from build123d import *

# Parameters (mm, degrees)
BOSS_EXTRUDE1_DEPTH = 3.1242
FILLET4_R           = 12.7
FILLET8_R           = 1.5875
FILLET9_R           = 3.175
CUT_EXTRUDE1_DEPTH  = 116.691473387
SKETCH3_R           = 1.5
CUT_EXTRUDE2_DEPTH  = 116.691473387


with BuildPart() as part:
    # Sketch1 → Boss-Extrude1 (new body)
    with BuildSketch(Plane.XY):
        Polygon((113.799832915, -6.443650697), (-97.791946085, -6.443650697), (-110.491946085, -0.093650697), (-110.491946085, 6.256349303), (-97.791946085, 22.131349303), (-91.441946085, 6.256349303), (113.799832915, 6.256349303), align=None)
        Polygon((-104.141946085, 6.256349303), (-99.460780317, 13.603434884), (-96.521946085, 6.256349303), align=None, mode=Mode.SUBTRACT)
    extrude(amount=BOSS_EXTRUDE1_DEPTH)

    # Fillet4
    fillet4_edges = [part.edges().sort_by_distance(p)[0] for p in [
        (-97.791946085, -6.443650697, 1.5621),
    ]]
    fillet(fillet4_edges, radius=FILLET4_R)

    # Fillet8
    fillet8_edges = [part.edges().sort_by_distance(p)[0] for p in [
        (-110.491946085, 6.256349303, 1.5621),
        (-97.791946085, 22.131349303, 1.5621),
        (-110.491946085, -0.093650697, 1.5621),
        (-104.141946085, 6.256349303, 1.5621),
        (-96.521946085, 6.256349303, 1.5621),
        (-99.460780317, 13.603434884, 1.5621),
    ]]
    fillet(fillet8_edges, radius=FILLET8_R)

    # Fillet9
    fillet9_edges = [part.edges().sort_by_distance(p)[0] for p in [
        (-91.441946085, 6.256349303, 1.5621),
    ]]
    fillet(fillet9_edges, radius=FILLET9_R)

    # Sketch2 → Cut-Extrude1 (cut, through all)
    with BuildSketch(Plane.XY.offset(3.1242)):
        with BuildLine():
            Line((-18.407167085, 2.38125), (-12.057167085, 2.38125))
            ThreePointArc((-12.057167085, 2.38125), (-9.675917085, 0), (-12.057167085, -2.38125))
            Line((-12.057167085, -2.38125), (-18.407167085, -2.38125))
            ThreePointArc((-18.407167085, -2.38125), (-20.788417085, 0), (-18.407167085, 2.38125))
        make_face()
    extrude(amount=-CUT_EXTRUDE1_DEPTH, mode=Mode.SUBTRACT)

    # Sketch3 → Cut-Extrude2 (cut, through all)
    with BuildSketch(Plane.XY.offset(3.1242)):
        with Locations((85.859832915, 3.716349303)):
            Circle(SKETCH3_R)
        with Locations((-89.400167085, 3.716349303)):
            Circle(SKETCH3_R)
    extrude(amount=-CUT_EXTRUDE2_DEPTH, mode=Mode.SUBTRACT)


solid = part.part
Read the model definition and answer for the solid it produces. Units are mm, in the model's axes. Coordinates: 2 decimals unless noted, no trailing zeros. Order: outer loops, then holes, each group sorted by start corner. A loop starts at its lowest first (then second) coordinate and runs counter-clockwise, first axis right, second up. Notation, with made-up numbers: (48, 43) -> (104, 43) arc R25 ccw to (104, 62) -> close; hole circle Ø5 at (82.5, -37.5). An arc over 180 degrees is marked (long way). Answer as a JSON object with one key per item and string values.
1) A cutting plane is placed at C-C, the plane y = 16.75. Determine the outline of the cut face in (x, z), plus the area to 3 significant figures.
Model answer:
{"outline": "(-102.1, 0) -> (-95.64, 0) -> (-95.64, 3.12) -> (-102.1, 3.12) -> close", "area": "20.2 mm²"}
2) Each of these flat-tipped pins is pushed along its axis until it touches: pin 1 (0.9 mm diameter, centred on x = -14.5, z = 2, fed in from +Y); pin 2 (1.2 mm diameter, centred on x = -99.5, z = 1.5, fed in from +Y); pin 3 (1 mm diameter, centred on y = 11, z = 0.5, fed in from -X). Where does it stop, or does it pass through?
Model answer:
{"pin 1": "stops at y = 6.26", "pin 2": "stops at y = 20.46", "pin 3": "stops at x = -107.1"}
3) A cutting plane is placed at B-B, the plane x = 15. Determine the outline of the cut face in (y, z).
Model answer:
{"outline": "(-6.44, 0) -> (6.26, 0) -> (6.26, 3.12) -> (-6.44, 3.12) -> close"}
4) A cutting plane is placed at A-A, the plane z = 0.6. State how many separate pieces and enclosed holes the cut face has, plus the area to 3 significant figures.
Model answer:
{"separate pieces": "1", "enclosed holes": "4", "area": "2,870 mm²"}
5) Consider line 1 along X through (y, z) = (4.25, 1.1); line 2 along Y through (x, z) = (22.5, 1.75); line 3 along X through (y, z) = (4.5, 2.7). Determine where each line is inside the solid, lowest interval first. Write a range as from..to.
Model answer:
{"line 1": "x = -110.49..-90.8, -88..84.46, 87.26..113.8", "line 2": "y = -6.44..6.26", "line 3": "x = -110.49..-90.68, -88.12..84.58, 87.14..113.8"}
